CAD build for the part. Positions are in the model's coordinates, mm. A direction names the side the tool comes from. Coordinates: 2 decimals unless noted, no trailing zeros. Order: outer loops, then holes, each group sorted by start corner. A loop starts at its lowest first (then second) coordinate and runs counter-clockwise, first axis right, second up. Notation, with made-up numbers: (52.5, -7) - (105.5, -7) arc R23 ccw to (105.5, 25) - close; hole circle Ø7 at (84.25, 14.25). An arc over 180 degrees is marked (long way). Use one line per item in the form item = value.
```python
from build123d import *

# Parameters (mm, degrees)
SKETCH1_R                = 0.95
BOSS_EXTRUDE1_DEPTH      = 2.625
SKETCH3_W                = 38
SKETCH3_H                = 2.75
CUT_EXTRUDE1_DEPTH       = 5
BOSS_EXTRUDE3_DEPTH      = 1.375
BOSS_EXTRUDE3_DEPTH_BACK = 2.625


with BuildPart() as part:
    # Sketch1 → Boss-Extrude1 (new, symmetric)
    with BuildSketch(Plane(origin=(0, 0, 0), x_dir=(1, 0, 0), z_dir=(0, 1, 0))):
        with BuildLine():
            Line((-0.393995074, 3.318856737), (-17.15759803, 1.993781046))
            ThreePointArc((-17.15759803, 1.993781046), (-19, 0), (-17.15759803, -1.993781046))
            Line((-17.15759803, -1.993781046), (-0.382476184, -4.590787721))
            ThreePointArc((-0.382476184, -4.590787721), (0, -4.620218562), (0.382476184, -4.590787721))
            Line((0.382476184, -4.590787721), (17.15759803, -1.993781046))
            ThreePointArc((17.15759803, -1.993781046), (19, 0), (17.15759803, 1.993781046))
            Line((17.15759803, 1.993781046), (0.393995074, 3.318856737))
            ThreePointArc((0.393995074, 3.318856737), (0, 3.334404121), (-0.393995074, 3.318856737))
        make_face()
        with Locations(Location((-17, 0, 0), (0, 0, 90))):
            Circle(SKETCH1_R, mode=Mode.SUBTRACT)
        with Locations(Location((17, 0, 0), (0, 0, 90))):
            Circle(SKETCH1_R, mode=Mode.SUBTRACT)
        with Locations(Location((0, -1.75, 0), (0, 0, 90))):
            Circle(SKETCH1_R, mode=Mode.SUBTRACT)
    extrude(amount=BOSS_EXTRUDE1_DEPTH, both=True)

    # Sketch3 → Cut-Extrude1 (cut, symmetric)
    with BuildSketch(Plane.XY):
        Rectangle(SKETCH3_W, SKETCH3_H)
    extrude(amount=CUT_EXTRUDE1_DEPTH, both=True, mode=Mode.SUBTRACT)


with BuildPart() as cut_extrude1_piece_1:
    # of the separate pieces the step leaves, piece 1, a body of its own (cut_extrude1_pieces)
    add(part.part.solids().sort_by_distance((0.393995074, -1.375, -3.318856737))[0])



with BuildPart() as cut_extrude1_piece_2:
    # of the separate pieces the step leaves, piece 2, a body of its own (cut_extrude1_pieces)
    add(part.part.solids().sort_by_distance((0.393995074, 2.625, -3.318856737))[0])


with BuildPart() as cut_extrude1_piece_1_1:
    add(cut_extrude1_piece_1.part)

    add(cut_extrude1_piece_2.part)  # Boss-Extrude3 merges Cut-Extrude1 piece 2
    # Sketch4 → Boss-Extrude3 (add, two sides: drawn at the far end of the back side and taken through both)
    with BuildSketch(Plane(origin=(0, 0, 0), x_dir=(1, 0, 0), z_dir=(0, 1, 0)).offset(-BOSS_EXTRUDE3_DEPTH_BACK)):
        with BuildLine():
            Line((6.699698425, -1.933474209), (11.720961536, 0.969441011))
            ThreePointArc((11.720961536, 0.969441011), (12.540704122, 0.750301575), (12.321564685, -0.069441011))
            Line((12.321564685, -0.069441011), (7.300301575, -2.972356232))
            ThreePointArc((7.300301575, -2.972356232), (6.480558989, -2.753216795), (6.699698425, -1.933474209))
        make_face()
    extrude(amount=BOSS_EXTRUDE3_DEPTH + BOSS_EXTRUDE3_DEPTH_BACK)


solid = cut_extrude1_piece_1_1.part
```
Item 1: Drill centre lines: line 1 (Y direction, x = -0.5, z = 2.75) (3 decimals); line 2 (Z direction, x = 17, y = 1.9); line 3 (X direction, y = 0.55, z = 1.25). Where is each one in solid material? Low to high. Write a range as [from, to].
Derived:
line_1 = [-2.625, -1.375], [1.375, 2.625]
line_2 = [-2.01, -0.95], [0.95, 2.02]
line_3 = [7.88, 10.28]
Item 2: Drop flat-ended pins along their axis: pin 1 (1.7 mm diameter, centred on x = 0, z = 1.75, fed in from +Y); pin 2 (2 mm diameter, centred on x = 17, z = 0, fed in from +Y) (3 decimals). Give the stop position or say it passes through.
Derived:
pin_1 = through
pin_2 = 2.625
Item 3: Cut at C-C, the plane x = -14.5. Write the cut outline in (y, z) (3 decimals).
Derived:
outline = (-2.625, -2.204) - (-1.375, -2.204) - (-1.375, 2.405) - (-2.625, 2.405) - close; (1.375, -2.204) - (2.625, -2.204) - (2.625, 2.405) - (1.375, 2.405) - close
Item 4: Cut at B-B, the plane y = -2.2. Write the cut outline in (x, z).
Derived:
outline = (-17.16, -1.99) - (-0.39, -3.32) arc R5 ccw to (0.39, -3.32) - (17.16, -1.99) arc R2 ccw to (17.16, 1.99) - (0.38, 4.59) arc R2.5 ccw to (-0.38, 4.59) - (-17.16, 1.99) arc R2 ccw to start; hole circle Ø1.9 at (-17, 0); hole circle Ø1.9 at (0, 1.75); hole circle Ø1.9 at (17, 0)
Item 5: 3-axis set-ups, long thin cutter, end or side, ignore diameter. For faces 1 (the face through (9.18, -0.02, 0.5)), 2 (the face through (12.534, -0.019, -0.762)), 3 (the face through (-8.887, -1.991, 3.274)): which of +Z, -Z, +X, -X, +Y, -Y reach the whole face in a straight line?
Derived:
face_1 = -Z, -X
face_2 = none
face_3 = +Z, -X, +Y, -Y
Item 6: Two-plate mould, pull along X, no slides. Class faces 4 (the face through (6.487, -0.019, 2.765)), 5 (the face through (-8.658, -1.991, -2.666)), 6 (the face through (0.58, -2.01, 2.5)): +X half, -X half, draft (parallel to the pull), parting line (faces both ways), or undercut.
Derived:
face_4 = parting line
face_5 = -X half
face_6 = undercut
Item 7: Cut at A-A, the plane x = 0. Write the cut outline in (y, z) (3 decimals), plus the area to 3 significant figures.
Derived:
outline = (-2.625, -3.334) - (-1.375, -3.334) - (-1.375, 0.8) - (-2.625, 0.8) - close; (-2.625, 2.7) - (-1.375, 2.7) - (-1.375, 4.62) - (-2.625, 4.62) - close; (1.375, -3.334) - (2.625, -3.334) - (2.625, 0.8) - (1.375, 0.8) - close; (1.375, 2.7) - (2.625, 2.7) - (2.625, 4.62) - (1.375, 4.62) - close
area = 15.1 mm²
Item 8: Cut at D-D, the plane z = 3.75. Write the cut outline in (x, y) (3 decimals).
Derived:
outline = (-5.813, -2.625) - (5.813, -2.625) - (5.813, -1.375) - (-5.813, -1.375) - close; (-5.813, 1.375) - (5.813, 1.375) - (5.813, 2.625) - (-5.813, 2.625) - close
